```python
from build123d import *

# Parameters (mm, degrees)
ESBO_O1_W                = 43
ESBO_O1_H                = 47
RESSALTO_EXTRUS_O1_DEPTH = 3
ESBO_O2_W                = 43
ESBO_O2_H                = 3
RESSALTO_EXTRUS_O2_DEPTH = 46
ESBO_O3_R                = 1.75
CORTE_EXTRUS_O1_DEPTH    = 56.950871307
ESBO_O4_R                = 1.75
CORTE_EXTRUS_O2_DEPTH    = 72.219730412
RESSALTO_EXTRUS_O3_DEPTH = 3
RESSALTO_EXTRUS_O4_DEPTH = 3
ESBO_O7_R                = 4
CORTE_EXTRUS_O3_DEPTH    = 3
FILETE1_R                = 3.5
FILETE2_R                = 7
FILETE3_R                = 3.5
FILETE4_R                = 5


with BuildPart() as part:
    # Esboço1 → Ressalto-extrusão1 (new body)
    with BuildSketch(Plane(origin=(0, 0, 0), x_dir=(1, 0, 0), z_dir=(0, 1, 0))):
        Rectangle(ESBO_O1_W, ESBO_O1_H)
    extrude(amount=RESSALTO_EXTRUS_O1_DEPTH)

    # Esboço2 → Ressalto-extrusão2 (add)
    with BuildSketch(Plane(origin=(0, 3, 0), x_dir=(1, 0, 0), z_dir=(0, 1, 0))):
        with Locations((0, -22)):
            Rectangle(ESBO_O2_W, ESBO_O2_H)
    extrude(amount=RESSALTO_EXTRUS_O2_DEPTH)

    # Esboço3 → Corte-extrusão1 (cut, through all)
    with BuildSketch(Plane(origin=(0, 3, 0), x_dir=(1, 0, 0), z_dir=(0, 1, 0))):
        with Locations(Location((14.945, 12.03, 0), (0, 0, 270))):
            Circle(ESBO_O3_R)
        with Locations(Location((14.945, -12.03, 0), (0, 0, 90))):
            Circle(ESBO_O3_R)
        with Locations(Location((-14.945, -12.03, 0), (0, 0, 270))):
            Circle(ESBO_O3_R)
        with Locations(Location((-14.945, 12.03, 0), (0, 0, 90))):
            Circle(ESBO_O3_R)
    extrude(amount=-CORTE_EXTRUS_O1_DEPTH, mode=Mode.SUBTRACT)

    # Esboço4 → Corte-extrusão2 (cut, through all)
    with BuildSketch(Plane.XY.offset(23.5)):
        with Locations((-15.5, 43)):
            Circle(ESBO_O4_R)
        with Locations((15.5, 43)):
            Circle(ESBO_O4_R)
        with Locations((-15.5, 12)):
            Circle(ESBO_O4_R)
        with Locations((15.5, 12)):
            Circle(ESBO_O4_R)
    extrude(amount=-CORTE_EXTRUS_O2_DEPTH, mode=Mode.SUBTRACT)

    # Esboço5 → Ressalto-extrusão3 (add)
    with BuildSketch(Plane.ZY.offset(21.5)):
        Polygon((-23.5, 0), (-23.5, 3), (20.5, 49), (23.5, 49), (23.5, 0), align=None)
    extrude(amount=RESSALTO_EXTRUS_O3_DEPTH)

    # Esboço6 → Ressalto-extrusão4 (add)
    with BuildSketch(Plane(origin=(21.5, 0, 0), x_dir=(0, 0, -1), z_dir=(1, 0, 0))):
        Polygon((23.5, 0), (-23.5, 0), (-23.5, 49), (-20.5, 49), (23.5, 3), align=None)
    extrude(amount=RESSALTO_EXTRUS_O4_DEPTH)

    # Esboço7 → Corte-extrusão3 (cut)
    with BuildSketch(Plane.XY.offset(23.5)):
        with Locations((0, 27.5)):
            Circle(ESBO_O7_R)
    extrude(amount=-CORTE_EXTRUS_O3_DEPTH, mode=Mode.SUBTRACT)

    # Filete1
    # the kernel refuses this fillet: 3.5 mm, written as the material it takes off along each edge
    with BuildSketch(Plane(origin=(-24.5, 49, 11.75), x_dir=(1, 0, 0), z_dir=(0, 0, 1)), Plane(origin=(24.5, 49, 32.25), x_dir=(-1, 0, 0), z_dir=(0, 0, -1))) as filete1_piece_1:
        with BuildLine():
            CenterArc((FILETE1_R, -FILETE1_R), FILETE1_R, 90, 90)
            Line((0, -FILETE1_R), (0, 0))
            Line((0, 0), (FILETE1_R, 0))
        make_face()
    extrude(amount=20.5, mode=Mode.SUBTRACT)

    # Filete2
    filete2_edges = [part.edges().sort_by_distance(p)[0] for p in [
        (0, 0, 23.5),
    ]]
    fillet(filete2_edges, radius=FILETE2_R)

    # Filete3
    # the kernel refuses this fillet: 3.5 mm, written as the material it takes off along each edge
    with BuildSketch(Plane(origin=(-24.5, -8.75, -23.5), x_dir=(0, 0, 1), z_dir=(0, 1, 0)), Plane(origin=(24.5, 11.75, -23.5), x_dir=(0, 0, 1), z_dir=(0, -1, 0))) as filete3_piece_1:
        with BuildLine():
            CenterArc((FILETE3_R, FILETE3_R), FILETE3_R, 180, 90)
            Line((0, FILETE3_R), (0, 0))
            Line((0, 0), (FILETE3_R, 0))
        make_face()
    extrude(amount=20.5, mode=Mode.SUBTRACT)

    # Filete4
    filete4_edges = [part.edges().sort_by_distance(p)[0] for p in [
        (0, 3, 20.5),
    ]]
    fillet(filete4_edges, radius=FILETE4_R)


solid = part.part
```
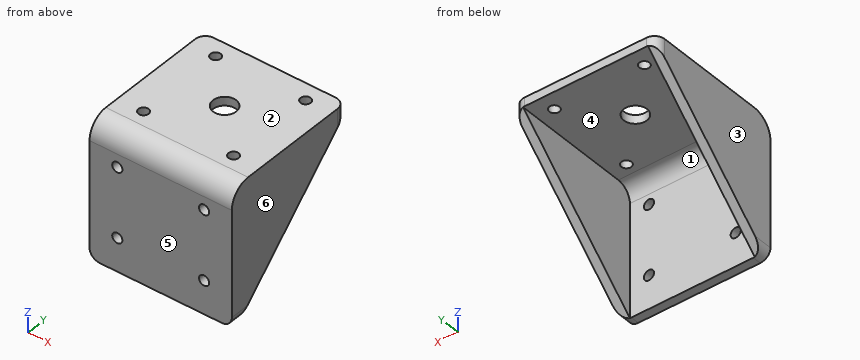
Design review of the part built by this model. Coordinates are the model's own, in mm. Face numbers are marked on the shaded views. A direction names the side the tool comes from. Coordinates: 2 decimals unless noted, no trailing zeros. Loops run counter-clockwise (first coordinate to the right, second up) from the corner with the lowest first, then second, coordinate; pieces in that order, holes last. Notation, with made-up numbers: (-35, -0.75) - (-12, -0.75) arc R19 ccw to (-12, 28.25) - close; hole circle Ø5 at (-4, -7). An arc over 180 degrees is marked (long way). Use CSV: the item, a comma, the result in double quotes. Start each with the question number.
1) The part is to be moulded in two halves that separate along X. For the marked faces 3, 4, 5 and 6, say which applies: +X half, -X half, draft (parallel to the pull), parting line (faces both ways), or undercut.
2) Consider section A-A on x = 0. Write out the cut boundary in (y, z), then the cut area to 3 significant figures.
3) Consider section C-C on z = -1.5. Write out the cut boundary in (x, y), then the cut area to 3 significant figures.
4) Consider section B-B on y = 37.5. Write out the cut boundary in (x, z).
5) Wall thickness on L1, parallel to X at y = 1.8, z = 12.03 (3 decimals); L2, parallel to X at y = 22, z = 19; L3, parallel to Y at x = 15, z = 21: over which ranges is each line inside the solid? List them lowest first. Write a range as from..to.
6) Tool access review of the marked faces 1 and 2: name each direction out of +Z, -Z, +X, -X, +Y, -Y from which nothing blocks a thin tool from reaching the whole face with its end or side.
7) Consider section D-D on z = 12.03. Write out the cut boundary in (x, y) (3 decimals).
8) For pin 1 Ø1 at (x, z) = (11, -6) entering from +Y; pin 2 Ø5 at (x, y) = (6, 29.5) entering from -Z, all flat-tipped, find the tip position at first contact; note any pin that passes through.
Geometry says:
1,face 3,"-X half"
1,face 4,"undercut"
1,face 5,"draft"
1,face 6,"+X half"
2,outline,"(0, -23.5) - (3, -23.5) - (3, 15.5) arc R5 cw to (8, 20.5) - (23.5, 20.5) - (23.5, 23.5) - (7, 23.5) arc R7 ccw to (0, 16.5) - close; (31.5, 20.5) - (49, 20.5) - (49, 23.5) - (31.5, 23.5) - close"
2,area,"250 mm^2"
3,outline,"(-24.5, 0) - (24.5, 0) - (24.5, 26) - (21.5, 26) - (21.5, 3) - (-21.5, 3) - (-21.5, 26) - (-24.5, 26) - close"
3,area,"285 mm^2"
4,outline,"(-24.5, 9.5) - (-21.5, 9.5) - (-21.5, 20.5) - (21.5, 20.5) - (21.5, 9.5) - (24.5, 9.5) - (24.5, 23.5) - (-24.5, 23.5) - close"
5,L1,"-24.5..-16.695, -13.195..13.195, 16.695..24.5"
5,L2,"-24.5..-21.5, 21.5..24.5"
5,L3,"1.64..10.32, 13.68..41.32, 44.68..49"
6,face 1,"-Z, +Y"
6,face 2,"+Z, +X, -X, +Y, -Y"
7,outline,"(-24.5, 0) - (-16.695, 0) - (-16.695, 3) - (-21.5, 3) - (-21.5, 40.145) - (-24.5, 40.145) - close; (-13.195, 0) - (13.195, 0) - (13.195, 3) - (-13.195, 3) - close; (16.695, 0) - (24.5, 0) - (24.5, 40.145) - (21.5, 40.145) - (21.5, 3) - (16.695, 3) - close"
8,pin 1,"y = 3"
8,pin 2,"z = 20.5"
